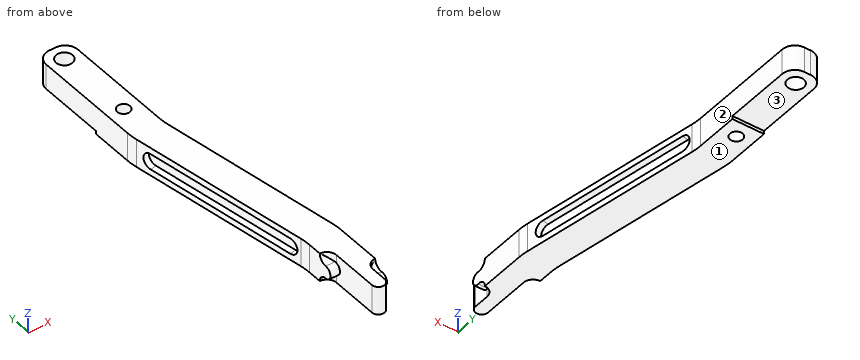
```python
from build123d import *

# Parameters (mm, degrees)
SKETCH1_R           = 2
SKETCH1_R_2         = 2.6
BOSS_EXTRUDE1_DEPTH = 9
FILLET1_R           = 4
SKETCH3_W           = 1
SKETCH3_H           = 25
CUT_EXTRUDE2_DEPTH  = 131.694299799
CUT_EXTRUDE3_DEPTH  = 132.837020597
BOSS_EXTRUDE2_DEPTH = 3
BOSS_EXTRUDE4_DEPTH = 5
CUT_EXTRUDE4_DEPTH  = 2
FILLET2_R           = 20
FILLET3_R           = 4


with BuildPart() as part:
    # Sketch1 → Boss-Extrude1 (new body)
    with BuildSketch(Plane.XY):
        Polygon((0, 0), (-10, 0), (-10, 30), (-20, 90), (-20, 130), (-10, 130), (-10, 90), (0, 30), align=None)
        with Locations((-15, 100)):
            Circle(SKETCH1_R, mode=Mode.SUBTRACT)
        with Locations((-15, 125)):
            Circle(SKETCH1_R_2, mode=Mode.SUBTRACT)
    extrude(amount=BOSS_EXTRUDE1_DEPTH)

    # Fillet1
    fillet1_edges = [part.edges().sort_by_distance(p)[0] for p in [
        (0, 0, 4.5),
        (-10, 0, 4.5),
    ]]
    fillet(fillet1_edges, radius=FILLET1_R)

    # Sketch3 → Cut-Extrude2 (cut, through all)
    with BuildSketch(Plane.ZY.offset(10)):
        with Locations((0.5, 117.5)):
            Rectangle(SKETCH3_W, SKETCH3_H)
    extrude(amount=CUT_EXTRUDE2_DEPTH, mode=Mode.SUBTRACT)

    # Sketch5 → Cut-Extrude3 (cut, through all)
    with BuildSketch(Plane.XY.offset(9)):
        with BuildLine():
            Line((-10, 4), (-10, 24))
            ThreePointArc((-10, 24), (-7.878679656, 23.121320344), (-7, 21))
            Line((-7, 21), (-7, 6))
            ThreePointArc((-7, 6), (-5, 4), (-3, 6))
            Line((-3, 6), (-3, 10.96659189))
            ThreePointArc((-3, 10.96659189), (-2.121320344, 13.087912234), (0, 13.96659189))
            Line((0, 13.96659189), (0, 4))
            ThreePointArc((0, 4), (-1.171572875, 1.171572875), (-4, 0))
            Line((-4, 0), (-6, 0))
            ThreePointArc((-6, 0), (-8.828427125, 1.171572875), (-10, 4))
        make_face()
    extrude(amount=-CUT_EXTRUDE3_DEPTH, mode=Mode.SUBTRACT)

    # Boss-Extrude2: read off the stored shape, not the designer's step
    # Boss-Extrude2 outline → Boss-Extrude2 (add)
    with BuildSketch(Plane.ZY):
        with BuildLine():
            Line((9, 13.96659189), (9, 30))
            Line((9, 30), (0, 30))
            Line((0, 30), (0, 13.96659189))
            Line((0, 13.96659189), (0.423395215, 13.96659189))
            ThreePointArc((0.423395215, 13.96659189), (2.009052541, 13.008624555), (2.499994655, 11.222291324))
            ThreePointArc((2.499994655, 11.222291324), (4.487608253, 9.000047793), (6.47522185, 11.222291324))
            ThreePointArc((6.47522185, 11.222291324), (6.966163965, 13.008624555), (8.551821291, 13.96659189))
            Line((8.551821291, 13.96659189), (9, 13.96659189))
        make_face()
    extrude(amount=BOSS_EXTRUDE2_DEPTH)

    # Sketch8 → Boss-Extrude4 (add)
    with BuildSketch(Plane.ZY.offset(10)):
        with BuildLine():
            Line((2.5, 21.5), (6.5, 21.5))
            ThreePointArc((6.5, 21.5), (4.5, 19.5), (2.5, 21.5))
        make_face()
        with BuildLine():
            ThreePointArc((0, 24), (1.767766953, 23.267766953), (2.5, 21.5))
            Line((2.5, 21.5), (6.5, 21.5))
            ThreePointArc((6.5, 21.5), (7.232233047, 23.267766953), (9, 24))
            Line((9, 24), (0, 24))
        make_face()
    extrude(amount=-BOSS_EXTRUDE4_DEPTH)

    # Sketch9 → Cut-Extrude4 (cut)
    with BuildSketch(Plane(origin=(4.931969619, 0.408182285, 0), x_dir=(0, 0, -1), z_dir=(0.9863939238321437, 0.16439898730535749, 0))):
        with BuildLine():
            Line((-7, 37), (-7, 85.827625303))
            ThreePointArc((-7, 85.827625303), (-4.5, 88.327625303), (-2, 85.827625303))
            Line((-2, 85.827625303), (-2, 37))
            ThreePointArc((-2, 37), (-4.5, 34.5), (-7, 37))
        make_face()
    cut_extrude4 = extrude(amount=-CUT_EXTRUDE4_DEPTH, mode=Mode.SUBTRACT)

    # Mirror1: Cut-Extrude4 across plane
    add(cut_extrude4.mirror(Plane(origin=(0, 0, 0), x_dir=(0, 0, 1), z_dir=(0.9863939238321437, 0.16439898730535743, 0))), mode=Mode.SUBTRACT)

    # Fillet2
    fillet2_edges = [part.edges().sort_by_distance(p)[0] for p in [
        (-10, 30, 4.5),
        (-20, 90, 4.5),
        (-10, 90, 4.5),
        (0, 30, 4.5),
    ]]
    fillet(fillet2_edges, radius=FILLET2_R)

    # Fillet3
    fillet3_edges = [part.edges().sort_by_distance(p)[0] for p in [
        (-20, 130, 5),
        (-10, 130, 5),
    ]]
    fillet(fillet3_edges, radius=FILLET3_R)


solid = part.part
```
Design review of the part built by this model. Coordinates are the model's own, in mm. Face numbers are marked on the shaded views. A direction names the side the tool comes from. Coordinates: 2 decimals unless noted, no trailing zeros. Loops run counter-clockwise (first coordinate to the right, second up) from the corner with the lowest first, then second, coordinate; pieces in that order, holes last. Notation, with made-up numbers: (28.5, 2.5) -> (53.5, 2.5) arc R22 ccw to (53.5, 32.5) -> close; hole circle Ø3 at (47, 33.25). An arc over 180 degrees is marked (long way). Answer as a JSON object with one key per item and string values.
Q1. Take a section at D-D on y = 26. Give the boundary of the cut face in (x, z), plus the area to 3 significant figures.
Answer block:
{"outline": "(-10, 0) -> (0, 0) -> (0, 9) -> (-10, 9) -> close", "area": "90.0 mm^2"}
Q2. Take a section at B-B on z = 5. Give the boundary of the cut face in (x, y), plus the area to 3 significant figures.
Answer block:
{"outline": "(-20, 91.66) arc R20 ccw to (-19.73, 88.37) -> (-19.31, 85.86) -> (-17.34, 86.19) -> (-8.51, 33.2) -> (-10.48, 32.87) -> (-10.27, 31.63) arc R20 cw to (-10, 28.34) -> (-10, 19.56) -> (-7, 19.56) -> (-7, 6) arc R2 ccw to (-3, 6) -> (-3, 9.07) -> (0, 9.07) -> (0, 28.34) arc R20 ccw to (-0.27, 31.63) -> (-0.75, 34.49) -> (-2.72, 34.16) -> (-11.55, 87.16) -> (-9.58, 87.48) -> (-9.73, 88.37) arc R20 cw to (-10, 91.66) -> (-10, 126) arc R4 ccw to (-14, 130) -> (-16, 130) arc R4 ccw to (-20, 126) -> close; hole circle Ø5.2 at (-15, 125); hole circle Ø4 at (-15, 100)", "area": "941 mm^2"}
Q3. Take a section at A-A on y = 100. Give the boundary of the cut face in (x, z), plus the area to 3 significant figures.
Answer block:
{"outline": "(-20, 0) -> (-17, 0) -> (-17, 9) -> (-20, 9) -> close; (-13, 0) -> (-10, 0) -> (-10, 9) -> (-13, 9) -> close", "area": "54.0 mm^2"}
Q4. Clearance check with flat-ended pins moving along their axes: pin 1 Ø1.5 at (y, z) = (8.5, 4.5) entering from +X; pin 2 Ø2.5 at (y, z) = (23.5, 2.5) entering from -X; pin 3 Ø4.5 at (y, z) = (15.5, 4.5) entering from -X; pin 4 Ø8 at (x, y) = (-14, 116) entering from -Z. State where each tip first meets the part, or that it passes through.
Answer block:
{"pin 1": "stops at x = 0", "pin 2": "stops at x = -10", "pin 3": "stops at x = -7", "pin 4": "stops at z = 1"}
Q5. To check wall thickness, follow L1, parallel to Z at x = -13.5, y = 58; L2, parallel to X at y = 125, z = 5; L3, parallel to Z at x = -16.75, y = 109.5. State the ranges of each line that lie inside material, in increasing order.
Answer block:
{"L1": "z = 0 to 2, 7 to 9", "L2": "x = -20 to -17.6, -12.4 to -10", "L3": "z = 1 to 9"}
Q6. Take a section at C-C on x = -5. Give the boundary of the cut face in (y, z).
Answer block:
{"outline": "(4, 0) -> (60, 0) -> (60, 2) -> (47.83, 2) -> (47.83, 7) -> (60, 7) -> (60, 9) -> (4, 9) -> close"}
Q7. Tool access review of the marked faces 1, 2 and 3: name each direction out of +Z, -Z, +X, -X, +Y, -Y from which nothing blocks a thin tool from reaching the whole face with its end or side.
Answer block:
{"face 1": "-Z, +X, -X, +Y, -Y", "face 2": "+Z, -Z, +X, +Y", "face 3": "-Z, +X, -X, +Y"}
